```python
from build123d import *

# Parameters (mm, degrees)
SKETCH1_W                        = 92
SKETCH1_H                        = 171
BOSS_EXTRUDE1_DEPTH              = 10
FILLET1_R                        = 46
SKETCH3_R                        = 3.5
CUT_EXTRUDE1_DEPTH               = 100.127443223
SKETCH4_R                        = 6
CUT_EXTRUDE2_DEPTH               = 6
CIRPATTERN1_COUNT                = 6
SKETCH6_R                        = 12.5
CUT_EXTRUDE3_DEPTH               = 10
SKETCH7_R                        = 8
CUT_EXTRUDE4_DEPTH               = 100.127443223
TAP_DRILL_FOR_M10X1_5_TAP1_D     = 8.5
TAP_DRILL_FOR_M10X1_5_TAP1_DEPTH = 6
TAP_DRILL_FOR_M10X1_5_TAP1_TIP   = 4.25
CUT_EXTRUDE5_DEPTH               = 4
FILLET2_R                        = 1


with BuildPart() as part:
    # Sketch1 → Boss-Extrude1 (new, symmetric)
    with BuildSketch(Plane.XY):
        Rectangle(SKETCH1_W, SKETCH1_H)
    extrude(amount=BOSS_EXTRUDE1_DEPTH, both=True)

    # Fillet1
    fillet1_edges = [part.edges().sort_by_distance(p)[0] for p in [
        (46, 85.5, 0),
        (-46, 85.5, 0),
    ]]
    fillet(fillet1_edges, radius=FILLET1_R - 0.0001)  # a hair under: the kernel refuses the full size

    # Sketch3 → Cut-Extrude1 (cut, through all)
    with BuildSketch(Plane.XY.offset(10)):
        with Locations((0, 78.5)):
            Circle(SKETCH3_R)
    cut_extrude1 = extrude(amount=-CUT_EXTRUDE1_DEPTH, mode=Mode.SUBTRACT)

    # Sketch4 → Cut-Extrude2 (cut)
    with BuildSketch(Plane(origin=(0, 0, -10), x_dir=(-1, 0, 0), z_dir=(0, 0, -1))):
        with Locations((0, 78.5)):
            Circle(SKETCH4_R)
    cut_extrude2 = extrude(amount=-CUT_EXTRUDE2_DEPTH, mode=Mode.SUBTRACT)

    # CirPattern1: Cut-Extrude1, Cut-Extrude2 ×6 about axis
    cirpattern1_axis = Axis((0, 39.5, 0), (0, 0, 1))
    add([cut_extrude1.rotate(cirpattern1_axis, i * 360 / CIRPATTERN1_COUNT) for i in range(1, CIRPATTERN1_COUNT)], mode=Mode.SUBTRACT)
    add([cut_extrude2.rotate(cirpattern1_axis, i * 360 / CIRPATTERN1_COUNT) for i in range(1, CIRPATTERN1_COUNT)], mode=Mode.SUBTRACT)

    # Sketch6 → Cut-Extrude3 (cut)
    with BuildSketch(Plane.XY.offset(10)):
        with Locations((0, 39.5)):
            Circle(SKETCH6_R)
    extrude(amount=-CUT_EXTRUDE3_DEPTH, mode=Mode.SUBTRACT)

    # Sketch7 → Cut-Extrude4 (cut, through all)
    with BuildSketch(Plane.XY.offset(10)):
        with Locations((0, 39.5)):
            Circle(SKETCH7_R)
    extrude(amount=-CUT_EXTRUDE4_DEPTH, mode=Mode.SUBTRACT)

    # Tap Drill for M10x1.5 Tap1
    with Locations(Plane(origin=(0, -85.5, 0), x_dir=(-1, 0, 0), z_dir=(0, -1, 0))):
        with Locations((30, 0), (-30, 0)):
            Hole(TAP_DRILL_FOR_M10X1_5_TAP1_D / 2, depth=TAP_DRILL_FOR_M10X1_5_TAP1_DEPTH)
            with Locations((0, 0, -(TAP_DRILL_FOR_M10X1_5_TAP1_DEPTH + TAP_DRILL_FOR_M10X1_5_TAP1_TIP / 2))):  # 90° drill point
                Cone(0, TAP_DRILL_FOR_M10X1_5_TAP1_D / 2, TAP_DRILL_FOR_M10X1_5_TAP1_TIP, mode=Mode.SUBTRACT)

    # Sketch12 → Cut-Extrude5 (cut)
    with BuildSketch(Plane.XY.offset(10)):
        with BuildLine():
            Line((34, -67.5), (34, -11.293700397))
            ThreePointArc((34, -11.293700397), (31.051285766, -6.127497229), (25.103448276, -6.039179666))
            ThreePointArc((25.103448276, -6.039179666), (0, -12.5), (-25.103448276, -6.039179666))
            ThreePointArc((-25.103448276, -6.039179666), (-31.051285766, -6.127497229), (-34, -11.293700397))
            Line((-34, -11.293700397), (-34, -67.5))
            ThreePointArc((-34, -67.5), (-32.242640687, -71.742640687), (-28, -73.5))
            Line((-28, -73.5), (28, -73.5))
            ThreePointArc((28, -73.5), (32.242640687, -71.742640687), (34, -67.5))
        make_face()
    cut_extrude5 = extrude(amount=-CUT_EXTRUDE5_DEPTH, mode=Mode.SUBTRACT)

    # Mirror1: Cut-Extrude5 across plane
    add(cut_extrude5.mirror(Plane.XY), mode=Mode.SUBTRACT)

    # Fillet2
    fillet2_edges = [part.edges().sort_by_distance(p)[0] for p in [
        (32.242640687, -71.742640687, 6),
        (0, -73.5, 6),
        (-32.242640687, -71.742640687, 6),
        (-34, -39.396850198, 6),
        (-31.051285766, -6.127497229, 6),
        (0, -12.5, 6),
        (31.051285766, -6.127497229, 6),
        (34, -39.396850198, 6),
        (32.242640687, -71.742640687, -6),
        (34, -39.396850198, -6),
        (31.051285766, -6.127497229, -6),
        (0, -12.5, -6),
        (-31.051285766, -6.127497229, -6),
        (-34, -39.396850198, -6),
        (-32.242640687, -71.742640687, -6),
        (0, -73.5, -6),
    ]]
    fillet(fillet2_edges, radius=FILLET2_R)


solid = part.part
```
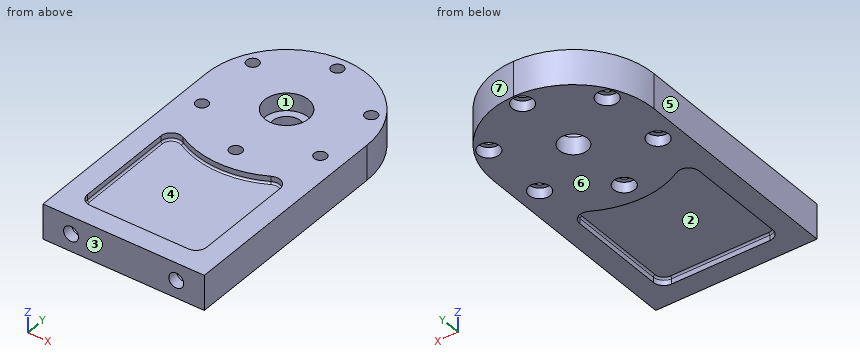
Verification items for the finished model (mm, model axes). Face numbers are marked on the shaded views. A direction names the side the tool comes from. Round coordinates to 2 decimals unless told otherwise and drop trailing zeros. Order: outer loops, then holes, each group sorted by start corner. A loop starts at its lowest first (then second) coordinate and runs counter-clockwise, first axis right, second up. Notation, with made-up numbers: (60.5, -34) -> (118.5, -34) arc R27 ccw to (118.5, -4) -> close; hole circle Ø11 at (-1, -20). An arc over 180 degrees is marked (long way). Put each result on its own line as item: value. Start each with the question number.
(1) Section check B-B (y = -34.5). Enter the section's corners in (x, z), then the cut area to 3 significant figures.
(2) Draft check along X on the marked faces 4, 5, 6 and 7. Enter one of: +X half, -X half, draft (parallel to the pull), parting line (faces both ways), or undercut.
(3) Depth check by flat-ended pin: pin 1 Ø6.5 at (x, y) = (-33.77, 59) entering from +Z; pin 2 Ø10 at (x, z) = (1, -3.5) entering from +Y; pin 3 Ø4 at (x, z) = (-12, 2) entering from +Y; pin 4 Ø9 at (x, y) = (33.77, 20) entering from -Z. Enter the tip coordinate at first touch or a pass-through.
(4) Section check A-A (y = 0.5). Enter the section's corners in (x, z).
(5) Section check C-C (y = 78.5). Enter the section's corners in (x, z).
(6) Tool access check on the marked faces 1, 2 and 3. Record the directions out of +Z, -Z, +X, -X, +Y, -Y that give a thin tool (end or side, any length) a straight path to the whole face; none if there is none.
(7) Material ranges on line 1 along Y through (x, z) = (0.5, 5.5); line 2 along Y through (x, z) = (-32.5, 7.25); line 3 along X through (y, z) = (-50, 9), recorded low to high.
Completed:
1. outline: (-46, -10) -> (-34, -10) -> (-34, -7) arc R1 cw to (-33, -6) -> (33, -6) arc R1 cw to (34, -7) -> (34, -10) -> (46, -10) -> (46, 10) -> (34, 10) -> (34, 7) arc R1 cw to (33, 6) -> (-33, 6) arc R1 cw to (-34, 7) -> (-34, 10) -> (-46, 10) -> close
1. area: 1,300 mm2
2. face 4: undercut
2. face 5: -X half
2. face 6: draft
2. face 7: +X half
3. pin 1: passes through
3. pin 2: stops at y = 85.5
3. pin 3: stops at y = 84.4
3. pin 4: stops at z = -4
4. outline: (-46, -10) -> (-6, -10) -> (-6, -4) -> (-3.5, -4) -> (-3.5, 10) -> (-46, 10) -> close; (3.5, -4) -> (6, -4) -> (6, -10) -> (46, -10) -> (46, 10) -> (3.5, 10) -> close
5. outline: (-24.39, -10) -> (-6, -10) -> (-6, -4) -> (-3.5, -4) -> (-3.5, 10) -> (-24.39, 10) -> close; (3.5, -4) -> (6, -4) -> (6, -10) -> (24.39, -10) -> (24.39, 10) -> (3.5, 10) -> close
6. face 1: +Z
6. face 2: -Z
6. face 3: +Z, -Z, +X, -X, -Y
7. line 1: y = -85.5 to -2.96, 3.96 to 27.01, 51.99 to 75.04, 81.96 to 85.5
7. line 2: y = -85.5 to -71.47, -7.33 to 16.74, 23.26 to 55.74, 62.26 to 72.05
7. line 3: x = -46 to -34, 34 to 46
